```python
from build123d import *

# Parameters (mm, degrees)
F1_DEPTH = 10


with BuildPart() as f1:
    # F0 (on Front) → F1 (new body)
    with BuildSketch(Plane.XZ):
        with BuildLine():
            ThreePointArc((-35.581168, -116.657823), (56.493287, -65.216884), (-10.920648, 15.895611))
            Line((-10.920648, 15.895611), (-33.676889, 15.895611))
            ThreePointArc((-33.676889, 15.895611), (-42.430831, 7.141669), (-33.676889, -1.612273))
            Line((-33.676889, -1.612273), (-29.301442, -1.612273))
            Line((-29.301442, -1.612273), (-17.38406, -1.612273))
            Line((-17.38406, -1.612273), (-29.301442, 3.387727))
            Line((-29.301442, 3.387727), (-33.676889, 3.387727))
            ThreePointArc((-33.676889, 3.387727), (-37.430831, 7.141669), (-33.676889, 10.895611))
            Line((-33.676889, 10.895611), (-10.920648, 10.895611))
            ThreePointArc((-10.920648, 10.895611), (51.577633, -64.302366), (-33.782985, -111.992361))
            Line((-33.782985, -111.992361), (-44.337623, -111.992361))
            Line((-44.337623, -111.992361), (-35.581168, -116.657823))
        make_face()
    extrude(amount=F1_DEPTH)


solid = f1.part
```
Verification items for the finished model (mm, model axes). A direction names the side the tool comes from. Round coordinates to 2 decimals unless told otherwise and drop trailing zeros. Write each loop counter-clockwise with the first axis right and the second up, starting at its lowest first coordinate (ties: lowest second). Pieces come first, ordered by that corner, then holes. Notation, with made-up numbers: (-38.5, 11.25) - (-14.5, 11.25) arc R19 cw to (-14.5, 37.25) - close; hole circle Ø4 at (33.5, -15.75). An arc over 180 degrees is marked (long way). Answer as a JSON object with one key per item and string values. Group by question number.
Q1. Section check B-B, the plane x = 39. Enter the section's corners in (y, z), plus the area to 3 significant figures.
Q2. Tool access check on faces 4 (the cylindrical face through (-37.43, -4.93, 7.06)), 5 (the flat face through (-39, -5, -111.992)), 6 (the flat face through (52, 0, -37)). Record the directions out of +Z, -Z, +X, -X, +Y, -Y that give a thin tool (end or side, any length) a straight path to the whole face; none if there is none.
Q3. Section check D-D, the plane z = -49. Enter the section's corners in (x, y), plus the area to 3 significant figures.
Q4. Thickness scan on line 1 (Z direction, x = -23, y = -8.75); line 2 (Z direction, x = -18, y = -3.75); line 3 (Z direction, x = -13, y = -5.75). Record the ranges inside material, lowest first.
Q5. Go/stop test with flat-tipped pins: pin 1 Ø4 at (x, y) = (20.5, -6.5) entering from -Z; pin 2 Ø5 at (x, y) = (-39.5, -6.5) entering from +Z; pin 3 Ø3 at (x, y) = (-10, -4.5) entering from -Z. Record where each tip stops, or that it passes through.
Q6. Mould release check, pull along X, two halves, no side actions. Record for faces 1 (the flat face through (52, -10, -37)), 2 (the cylindrical face through (-42.43, -4.93, 7.33)), 3 (the flat face through (-22, -5, 10.896)): released by +X, released by -X, zero draft, split by the parting line, or undercut.
Q7. Section check A-A, the plane y = -3. Enter the section's corners in (x, z), plus the area to 3 significant figures.
Q8. Section check C-C, the plane x = 22. Enter the section's corners in (y, z).
Found:
{
 "1": {"outline": "(-10, -99.68) - (0, -99.68) - (0, -92.03) - (-10, -92.03) - close; (-10, -13.32) - (0, -13.32) - (0, -5.67) - (-10, -5.67) - close", "area": "153 mm^2"},
 "2": {"face 4": "+Y, -Y", "face 5": "-X, +Y, -Y", "face 6": "+Z, -Z, +X, -X, +Y"},
 "3": {"outline": "(52.54, -10) - (57.55, -10) - (57.55, 0) - (52.54, 0) - close", "area": "50.1 mm^2"},
 "4": {"line 1": "z = -120.17 to -115.09, -1.61 to 0.74, 10.9 to 15.9", "line 2": "z = -120.88 to -115.85, -1.61 to -1.35, 10.9 to 15.9", "line 3": "z = -121.21 to -116.21, 10.9 to 15.9"},
 "5": {"pin 1": "stops at z = -114.61", "pin 2": "stops at z = 15.24", "pin 3": "stops at z = -121.25"},
 "6": {"face 1": "zero draft", "face 2": "released by -X", "face 3": "undercut"},
 "7": {"outline": "(-44.34, -111.99) - (-35.58, -116.66) arc R68.57 ccw (long way) to (-10.92, 15.9) - (-33.68, 15.9) arc R8.75 ccw to (-33.68, -1.61) - (-17.38, -1.61) - (-29.3, 3.39) - (-33.68, 3.39) arc R3.75 cw to (-33.68, 10.9) - (-10.92, 10.9) arc R63.57 cw (long way) to (-33.78, -111.99) - close", "area": "1,450 mm^2"},
 "8": {"outline": "(-10, -112.83) - (0, -112.83) - (0, -107.06) - (-10, -107.06) - close; (-10, 1.71) - (0, 1.71) - (0, 7.48) - (-10, 7.48) - close"}
}
